For this review, take the finished solid that the model builds, in its own axes (mm). A direction names the side the tool comes from. Coordinates: 2 decimals unless noted, no trailing zeros. Write each loop counter-clockwise with the first axis right and the second up, starting at its lowest first coordinate (ties: lowest second). Pieces come first, ordered by that corner, then holes.
1) Insertion check: P1, Ø12, axis at x = -29.5, z = 11, coming from the -Y side; P2, Ø9, axis at x = -53, y = -24.5, coming from the -Z side; P3, Ø3, axis at x = 39.5, y = -4.5, coming from the +Z side. Each pin has a flat end and moves straight along its axis. Give the tip position at first contact, or say it passes through.
2) To check wall thickness, follow line 1 along Y through (x, z) = (15.5, 36); line 2 along X through (y, z) = (-23, 48); line 3 along Z through (x, y) = (-51.5, -19). State the ranges of each line that lie inside material, in increasing order.
3) We need section C-C on y = -18.5. Write out the cut boundary in (x, z).
4) We need section D-D on z = 33. Write out the cut boundary in (x, y), then the cut area to 3 significant figures.
5) Mouldability with a two-part tool opening along Z and no side actions: class faces 4 (the face through (-52, -18, -9.218)), 5 (the face through (23, -10, 15)), 6 (the face through (12, -5, 54.365)), 7 (the face through (-0.551, -4.93, -33.782)) as pulls with the +Z half, pulls with the -Z half, needs draft (parallel to the pull), parting line crosses it, or undercut.
6) For faces 1 (the face through (35.389, -5, 47)), 2 (the face through (-61.008, -13, 44)), 3 (the face through (-11.717, -5, 47)), list the 3-axis set-ups (+Z, -Z, +X, -X, +Y, -Y) from which the entire face can be reached by the end or side of a thin tool; tool diameter is ignored.
7) We need section B-B on x = -42. Write out the cut boundary in (y, z), then the cut area to 3 significant figures.
8) We need section A-A on z = 44. Write out the cut boundary in (x, y).
from build123d import *

# Parameters (mm, degrees)
F0_W     = 84.6221074462
F0_H     = 86.6273678839
F0_R     = 26.5937510692
F1_DEPTH = 10
F2_W     = 26.760289222
F2_H     = 48.1868900824
F2_W_2   = 10
F3_DEPTH = 30
F4_W     = 29.033318162
F4_H     = 15.370901674
F5_DEPTH = 25.4
F6_W     = 47.1061710268
F6_H     = 18.6824947596
F7_DEPTH = 10


with BuildPart() as f1:
    # F0 (on Front) → F1 (new body)
    with BuildSketch(Plane.XZ):
        with Locations((5.1468424499, -4.3447371572)):
            Rectangle(F0_W, F0_H)
        with Locations((5.2136839367, -7.8205261379)):
            Circle(F0_R, mode=Mode.SUBTRACT)
    extrude(amount=F1_DEPTH)

    # F2 (on face) → F3 (join)
    with BuildSketch(Plane(origin=(-37.1642112732, 0, 0), x_dir=(0, -1, 0), z_dir=(-1, 0, 0))):
        with Locations((23.380144611, 14.8755017435)):
            Rectangle(F2_W, F2_H)
        with Locations((5, 14.8755017435)):
            Rectangle(F2_W_2, F2_H)
    extrude(amount=F3_DEPTH)

    # F4 (on Front) → F5 (join)
    with BuildSketch(Plane.XZ):
        with Locations((-46.4909225702, 41.9942829758)):
            Rectangle(F4_W, F4_H)
    extrude(amount=F5_DEPTH)

    # F6 (on Front) → F7 (join)
    with BuildSketch(Plane.XZ):
        with Locations((11.8363192305, 45.0233183801)):
            Rectangle(F6_W, F6_H)
    extrude(amount=F7_DEPTH)


solid = f1.part
Result:
1. P1: stops at y = -10
1. P2: stops at z = -9.22
1. P3: stops at z = 38.97
2. line 1: y = -10 to 0
2. line 2: x = -61.01 to -31.97
2. line 3: z = -9.22 to 49.68
3. outline: (-67.16, -9.22) - (-37.16, -9.22) - (-37.16, 34.31) - (-31.97, 34.31) - (-31.97, 49.68) - (-61.01, 49.68) - (-61.01, 38.97) - (-67.16, 38.97) - close
4. outline: (-67.16, -36.76) - (-37.16, -36.76) - (-37.16, -10) - (47.46, -10) - (47.46, 0) - (-67.16, 0) - close
4. area: 1,950 mm2
5. face 4: pulls with the -Z half
5. face 5: needs draft
5. face 6: pulls with the +Z half
5. face 7: undercut
6. face 1: +Z, +X, +Y, -Y
6. face 2: +Z, -X, +Y, -Y
6. face 3: +Z, +Y, -Y
7. outline: (-36.76, -9.22) - (0, -9.22) - (0, 49.68) - (-25.4, 49.68) - (-25.4, 38.97) - (-36.76, 38.97) - close
7. area: 2,040 mm2
8. outline: (-61.01, -25.4) - (-31.97, -25.4) - (-31.97, 0) - (-61.01, 0) - close; (-11.72, -10) - (35.39, -10) - (35.39, 0) - (-11.72, 0) - close
